The listing builds one solid part. Answer for the finished solid, in the listing's coordinates (mm). Round coordinates to 2 decimals unless told otherwise and drop trailing zeros. Order: outer loops, then holes, each group sorted by start corner. A loop starts at its lowest first (then second) coordinate and runs counter-clockwise, first axis right, second up. Notation, with made-up numbers: (31, -12.5) -> (54, -12.5) arc R23 cw to (54, -4.5) -> close; hole circle Ø9 at (63, -17.5). An arc over 180 degrees is marked (long way). Return JSON: item names as keys, results as strings. Group by question number.
(1) The part is cut by section B-B (y = 2.3). Count the separate pieces of the cut face and the enclosed holes in it, plus the area to 3 significant figures.
(2) Consider line 1 (X direction, y = 2.7, z = -28); line 2 (X direction, y = 1.15, z = -18.5); line 3 (X direction, y = 2.5, z = -44.5). Determine where each line is inside the solid, lowest interval first. Write a range as [from, to].
(3) The part is cut by section A-A (x = 154.5). Determine the outline of the cut face in (y, z).
(4) This flat-tipped pin is pushed along its axis until it touches: pin 1 (1.2 mm diameter, centred on y = 2.5, z = -48.5, fed in from -X). Where does it stop, or does it pass through?
from build123d import *

# Parameters (mm, degrees)
SKETCH1_W           = 104
SKETCH1_H           = 57
SKETCH1_W_2         = 4
SKETCH1_H_2         = 10
BOSS_EXTRUDE1_DEPTH = 4


with BuildPart() as part:
    # Sketch1 → Boss-Extrude1 (new body)
    # profile 1 of 7: a face of its own
    with BuildSketch(Plane(origin=(0, 0, 0), x_dir=(1, 0, 0), z_dir=(0, 1, 0))):
        Polygon((0, 10), (0, 0), (200, 0), (200, 10), (200, 30), (200, 40), (200, 60), (200, 70), (0, 70), (0, 60), (0, 40), (0, 30), align=None)
        with BuildLine():
            ThreePointArc((35, 21), (36, 20), (35, 19))
            Line((35, 19), (15, 19))
            ThreePointArc((15, 19), (14, 20), (15, 21))
            Line((15, 21), (35, 21))
        make_face(mode=Mode.SUBTRACT)
        with BuildLine():
            ThreePointArc((35, 25), (36, 24), (35, 23))
            Line((35, 23), (15, 23))
            ThreePointArc((15, 23), (14, 24), (15, 25))
            Line((15, 25), (35, 25))
        make_face(mode=Mode.SUBTRACT)
        with BuildLine():
            ThreePointArc((35, 29), (36, 28), (35, 27))
            Line((35, 27), (15, 27))
            ThreePointArc((15, 27), (14, 28), (15, 29))
            Line((15, 29), (35, 29))
        make_face(mode=Mode.SUBTRACT)
        with BuildLine():
            ThreePointArc((35, 33), (36, 32), (35, 31))
            Line((35, 31), (15, 31))
            ThreePointArc((15, 31), (14, 32), (15, 33))
            Line((15, 33), (35, 33))
        make_face(mode=Mode.SUBTRACT)
        with BuildLine():
            ThreePointArc((60, 21), (61, 20), (60, 19))
            Line((60, 19), (40, 19))
            ThreePointArc((40, 19), (39, 20), (40, 21))
            Line((40, 21), (60, 21))
        make_face(mode=Mode.SUBTRACT)
        with BuildLine():
            ThreePointArc((60, 25), (61, 24), (60, 23))
            Line((60, 23), (40, 23))
            ThreePointArc((40, 23), (39, 24), (40, 25))
            Line((40, 25), (60, 25))
        make_face(mode=Mode.SUBTRACT)
        with BuildLine():
            ThreePointArc((60, 29), (61, 28), (60, 27))
            Line((60, 27), (40, 27))
            ThreePointArc((40, 27), (39, 28), (40, 29))
            Line((40, 29), (60, 29))
        make_face(mode=Mode.SUBTRACT)
        with BuildLine():
            ThreePointArc((60, 33), (61, 32), (60, 31))
            Line((60, 31), (40, 31))
            ThreePointArc((40, 31), (39, 32), (40, 33))
            Line((40, 33), (60, 33))
        make_face(mode=Mode.SUBTRACT)
        with BuildLine():
            ThreePointArc((35, 37), (36, 36), (35, 35))
            Line((35, 35), (15, 35))
            ThreePointArc((15, 35), (14, 36), (15, 37))
            Line((15, 37), (35, 37))
        make_face(mode=Mode.SUBTRACT)
        with BuildLine():
            ThreePointArc((35, 41), (36, 40), (35, 39))
            Line((35, 39), (15, 39))
            ThreePointArc((15, 39), (14, 40), (15, 41))
            Line((15, 41), (35, 41))
        make_face(mode=Mode.SUBTRACT)
        with BuildLine():
            ThreePointArc((35, 45), (36, 44), (35, 43))
            Line((35, 43), (15, 43))
            ThreePointArc((15, 43), (14, 44), (15, 45))
            Line((15, 45), (35, 45))
        make_face(mode=Mode.SUBTRACT)
        with BuildLine():
            ThreePointArc((35, 49), (36, 48), (35, 47))
            Line((35, 47), (15, 47))
            ThreePointArc((15, 47), (14, 48), (15, 49))
            Line((15, 49), (35, 49))
        make_face(mode=Mode.SUBTRACT)
        with BuildLine():
            ThreePointArc((35, 53), (36, 52), (35, 51))
            Line((35, 51), (15, 51))
            ThreePointArc((15, 51), (14, 52), (15, 53))
            Line((15, 53), (35, 53))
        make_face(mode=Mode.SUBTRACT)
        with BuildLine():
            ThreePointArc((60, 37), (61, 36), (60, 35))
            Line((60, 35), (40, 35))
            ThreePointArc((40, 35), (39, 36), (40, 37))
            Line((40, 37), (60, 37))
        make_face(mode=Mode.SUBTRACT)
        with BuildLine():
            ThreePointArc((60, 41), (61, 40), (60, 39))
            Line((60, 39), (40, 39))
            ThreePointArc((40, 39), (39, 40), (40, 41))
            Line((40, 41), (60, 41))
        make_face(mode=Mode.SUBTRACT)
        with BuildLine():
            ThreePointArc((60, 45), (61, 44), (60, 43))
            Line((60, 43), (40, 43))
            ThreePointArc((40, 43), (39, 44), (40, 45))
            Line((40, 45), (60, 45))
        make_face(mode=Mode.SUBTRACT)
        with BuildLine():
            ThreePointArc((60, 49), (61, 48), (60, 47))
            Line((60, 47), (40, 47))
            ThreePointArc((40, 47), (39, 48), (40, 49))
            Line((40, 49), (60, 49))
        make_face(mode=Mode.SUBTRACT)
        with BuildLine():
            ThreePointArc((60, 53), (61, 52), (60, 51))
            Line((60, 51), (40, 51))
            ThreePointArc((40, 51), (39, 52), (40, 53))
            Line((40, 53), (60, 53))
        make_face(mode=Mode.SUBTRACT)
        with Locations((132, 35)):
            Rectangle(SKETCH1_W, SKETCH1_H, mode=Mode.SUBTRACT)
    # profile 2 of 7: a face of its own
    with BuildSketch(Plane(origin=(0, 0, 0), x_dir=(1, 0, 0), z_dir=(0, 1, 0))):
        with Locations((-2, 5)):
            Rectangle(SKETCH1_W_2, SKETCH1_H_2)
    # profile 3 of 7: a face of its own
    with BuildSketch(Plane(origin=(0, 0, 0), x_dir=(1, 0, 0), z_dir=(0, 1, 0))):
        with Locations((202, 5)):
            Rectangle(SKETCH1_W_2, SKETCH1_H_2)
    # profile 4 of 7: a face of its own
    with BuildSketch(Plane(origin=(0, 0, 0), x_dir=(1, 0, 0), z_dir=(0, 1, 0))):
        with Locations((-2, 35)):
            Rectangle(SKETCH1_W_2, SKETCH1_H_2)
    # profile 5 of 7: a face of its own
    with BuildSketch(Plane(origin=(0, 0, 0), x_dir=(1, 0, 0), z_dir=(0, 1, 0))):
        with Locations((202, 35)):
            Rectangle(SKETCH1_W_2, SKETCH1_H_2)
    # profile 6 of 7: a face of its own
    with BuildSketch(Plane(origin=(0, 0, 0), x_dir=(1, 0, 0), z_dir=(0, 1, 0))):
        with Locations((-2, 65)):
            Rectangle(SKETCH1_W_2, SKETCH1_H_2)
    # profile 7 of 7: a face of its own
    with BuildSketch(Plane(origin=(0, 0, 0), x_dir=(1, 0, 0), z_dir=(0, 1, 0))):
        with Locations((202, 65)):
            Rectangle(SKETCH1_W_2, SKETCH1_H_2)
    extrude(amount=BOSS_EXTRUDE1_DEPTH)


solid = part.part
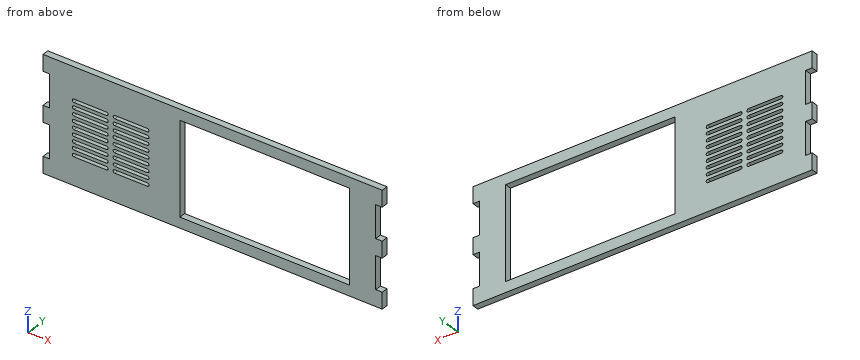
Answer below:
{
 "1": {"separate pieces": "1", "enclosed holes": "19", "area": "7,540 mm²"},
 "2": {"line 1": "x = [0, 14], [36, 39], [61, 80], [184, 200]", "line 2": "x = [0, 80], [184, 200]", "line 3": "x = [0, 14.13], [35.87, 39.13], [60.87, 80], [184, 200]"},
 "3": {"outline": "(0, -70) -> (4, -70) -> (4, -63.5) -> (0, -63.5) -> close; (0, -6.5) -> (4, -6.5) -> (4, 0) -> (0, 0) -> close"},
 "4": {"pin 1": "stops at x = 0"}
}
